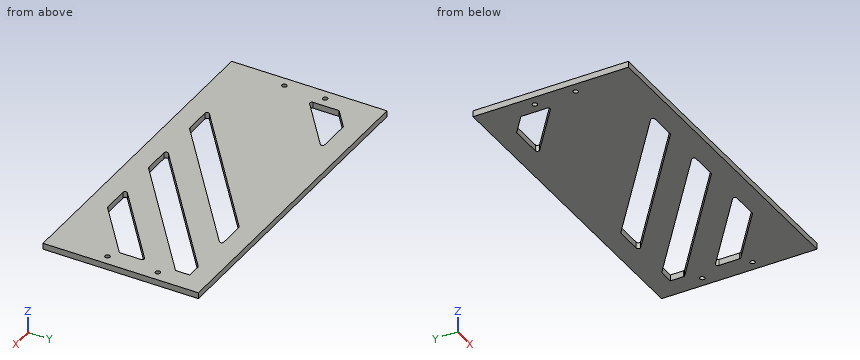
Autodesk Inventor part; units mm, degrees
ref_plane "YZ Plane" through (0, 0, 0) normal (1, 0, 0) x (0, 1, 0)
ref_plane "XZ Plane" through (0, 0, 0) normal (0, 1, 0) x (-1, 0, 0)
ref_plane "XY Plane" through (0, 0, 0) normal (0, 0, 1) x (1, 0, 0)
sketch "草图1" plane through (0, 0, 0) normal (0, 0, 1) x (1, 0, 0)
  line L0 (80.5, -38.1196) -> (-80.5, -38.1196)
  line L1 (-80.5, -38.1196) -> (-80.5, 38.1196)
  line L2 (-80.5, 38.1196) -> (80.5, 38.1196)
  line L3 (80.5, 38.1196) -> (80.5, -38.1196)
  line L4 (80.5, -38.1196) -> (-80.5, 38.1196) construction
  line L5 (-80.5, -38.1196) -> (80.5, 38.1196) construction
  point P0 (0, 0)
  dimension "d1" = 161
extrude "拉伸1" add sketch "草图1" along normal blind 3
sketch "草图2" plane through (0, 0, 3) normal (0, 0, 1) x (1, 0, 0)
  line L0 (61.6798, 137.1398) -> (-176.304, -50.1889)
  line L1 (-176.304, -50.1889) -> (-170.1188, -58.0466)
  line L2 (-170.1188, -58.0466) -> (67.865, 129.282)
  line L3 (67.865, 129.282) -> (61.6798, 137.1398)
  line L4 (80.5, 38.1196) -> (-80.5, 38.1196)
  line L5 (96.6798, 137.1398) -> (-141.304, -50.1889)
  line L6 (102.865, 129.282) -> (96.6798, 137.1398)
  line L7 (-135.1188, -58.0466) -> (102.865, 129.282)
  line L8 (-141.304, -50.1889) -> (-135.1188, -58.0466)
  line L9 (131.6798, 137.1398) -> (-106.304, -50.1889)
  line L10 (137.865, 129.282) -> (131.6798, 137.1398)
  line L11 (-100.1188, -58.0466) -> (137.865, 129.282)
  line L12 (-106.304, -50.1889) -> (-100.1188, -58.0466)
  line L13 (166.6798, 137.1398) -> (-71.304, -50.1889)
  line L14 (172.865, 129.282) -> (166.6798, 137.1398)
  line L15 (-65.1188, -58.0466) -> (172.865, 129.282)
  line L16 (-71.304, -50.1889) -> (-65.1188, -58.0466)
  line L17 (201.6798, 137.1398) -> (-36.304, -50.1889)
  line L18 (207.865, 129.282) -> (201.6798, 137.1398)
  line L19 (-30.1188, -58.0466) -> (207.865, 129.282)
  line L20 (-36.304, -50.1889) -> (-30.1188, -58.0466)
  line L21 (236.6798, 137.1398) -> (-1.304, -50.1889)
  line L22 (242.865, 129.282) -> (236.6798, 137.1398)
  line L23 (4.8812, -58.0466) -> (242.865, 129.282)
  line L24 (-1.304, -50.1889) -> (4.8812, -58.0466)
  line L25 (271.6798, 137.1398) -> (33.696, -50.1889)
  line L26 (277.865, 129.282) -> (271.6798, 137.1398)
  line L27 (39.8812, -58.0466) -> (277.865, 129.282)
  line L28 (33.696, -50.1889) -> (39.8812, -58.0466)
  line L29 (-80.5, 38.1196) -> (-80.5, -38.1196)
  line L30 (80.5, -38.1196) -> (80.5, 38.1196)
  line L31 (-80.5, -38.1196) -> (80.5, -38.1196)
  line L32 (-70.5, 28.1196) -> (70.5, 28.1196)
  line L33 (70.5, 28.1196) -> (70.5, -28.1196)
  line L34 (70.5, -28.1196) -> (-70.5, -28.1196)
  line L35 (-70.5, -28.1196) -> (-70.5, 28.1196)
  point P0 (0, 0)
  point P1 (-51.1269, 35.6177)
  point P2 (-16.1269, 35.6177)
  point P3 (18.8731, 35.6177)
  point P4 (53.8731, 35.6177)
  point P5 (88.8731, 35.6177)
  point P6 (123.8731, 35.6177)
  point P7 (158.8731, 35.6177)
  point P8 (26.733, -28.1196)
  point P9 (42.9006, -28.1196)
  point P10 (70.5, -6.3948)
  point P11 (70.5, 6.3315)
  point P12 (-8.267, -28.1196)
  point P13 (7.9006, -28.1196)
  point P14 (70.5, 21.1554)
  point P15 (63.1798, 28.1196)
  point P16 (-43.267, -28.1196)
  point P17 (-27.0994, -28.1196)
  point P18 (44.3475, 28.1196)
  point P19 (28.1798, 28.1196)
  point P20 (-70.5, -7.182)
  point P21 (-70.5, -22.0058)
  point P22 (-6.8202, 28.1196)
  point P23 (-25.6525, 28.1196)
  point P24 (-70.5, 20.3682)
  point P25 (-70.5, 5.5444)
  point P26 (-41.8202, 28.1196)
  point P27 (-60.6525, 28.1196)
  dimension "d5" = 10
  dimension "d8" = 35
  dimension "d13" = 10
extrude "拉伸2" cut sketch "草图2" against normal blind 10 contours L32 L5 L35 L2 | L32 L15 L34 L13 | L32 L33 L19 L34 L17 | L21 L33 L23 L34
fillet "圆角1" radius 1 14 edges at (28.1798, 28.1196, 1.5) (44.3475, 28.1196, 1.5) (63.1798, 28.1196, 1.5) (70.5, 21.1554, 1.5) (70.5, 6.3315, 1.5) (26.733, -28.1196, 1.5) (42.9006, -28.1196, 1.5) (70.5, -6.3948, 1.5) (-8.267, -28.1196, 1.5) (7.9006, -28.1196, 1.5) (-43.267, -28.1196, 1.5) (-27.0994, -28.1196, 1.5) (-70.5, 5.5444, 1.5) (-41.8202, 28.1196, 1.5)
sketch "草图3" plane through (0, 0, 3) normal (0, 0, 1) x (1, 0, 0)
  ellipse E0 centre (75.5, 15.3081) end of major axis (76.7, 15.3081) minor radius 1.1476
  circle A0 centre (75.5, -9.3544) radius 1.2
  circle A1 centre (-75.5, 10.6456) radius 1.2
  circle A2 centre (-75.5, -9.3544) radius 1.2
  point P0 (0, 0)
extrude "拉伸3" cut sketch "草图3" against normal blind 10
equation "\"d14\" = d5"
equation "\"d17\" = d5"
properties part number "后板2"
CAD build for the part. Positions are in the model's coordinates, mm. Round coordinates to 2 decimals unless told otherwise and drop trailing zeros. Loops run counter-clockwise (first coordinate to the right, second up) from the corner with the lowest first, then second, coordinate; pieces in that order, holes last. Notation, with made-up numbers: M 7.5,54 L 50.5,54 A19 cw 50.5,88 Z; hole C -6,-28 d2. An arc over 180 degrees is marked long. Use a Markdown table: item, result. Add a question column.
(1) Flat gauge pin, fed straight in: pin 1 (2 mm diameter, centred on x = -75.5, y = 10.65, fed in from -Z). Where does the tip first touch, or does it go through?
(2) Cut at A-A (x = -18). Give the cut face in (y, z), and give its area (3 significant figures).
(3) Cut at B-B (x = 61). Give the cut face in (y, z).
(4) Drill centre lines: line 1 (Y direction, x = -75.5, z = 2.45); line 2 (Y direction, x = 75.5, z = 1.3); line 3 (X direction, y = 13, z = 1.4). Where is each one in solid material? Low to high.
(5) Cut at D-D (z = 0.65). State how many separate pieces and enclosed holes the cut face has, and give its area (3 significant figures).
(6) Cut at C-C (x = 34). Give the cut face in (y, z), and give its area (3 significant figures).
Geometry says:
| question | item | result |
|---|---|---|
| 1 | pin 1 | passes through |
| 2 | outline | M -38.12,0 L -20.96,0 L -20.96,3 L -38.12,3 Z; M -8.23,0 L 38.12,0 L 38.12,3 L -8.23,3 Z |
| 2 | area | 191 mm² |
| 3 | outline | M -38.12,0 L -13.87,0 L -13.87,3 L -38.12,3 Z; M -1.15,0 L 13.68,0 L 13.68,3 L -1.15,3 Z; M 26.4,0 L 38.12,0 L 38.12,3 L 26.4,3 Z |
| 4 | line 1 | y = -38.12 to -10.55, -8.15 to 9.45, 11.85 to 38.12 |
| 4 | line 2 | y = -38.12 to -10.55, -8.15 to 14.16, 16.46 to 38.12 |
| 4 | line 3 | x = -80.5 to -70.5, -61.03 to 8.97, 25.14 to 43.97, 60.14 to 80.5 |
| 5 | separate pieces | 1 |
| 5 | enclosed holes | 8 |
| 5 | area | 9,740 mm² |
| 6 | outline | M -38.12,0 L -28.12,0 L -28.12,3 L -38.12,3 Z; M -22.4,0 L -7.58,0 L -7.58,3 L -22.4,3 Z; M 5.15,0 L 19.97,0 L 19.97,3 L 5.15,3 Z; M 28.12,0 L 38.12,0 L 38.12,3 L 28.12,3 Z |
| 6 | area | 149 mm² |
